from build123d import *

# Parameters (mm, degrees)
SKIZZE1_R                       = 32.5
SKIZZE1_R_2                     = 5
AUFSATZ_LINEAR_AUSTRAGEN1_DEPTH = 5
SCHNITT_LINEAR_AUSTRAGEN1_DEPTH = 6
KREISMUSTER1_COUNT              = 8


with BuildPart() as part:
    # Skizze1 → Aufsatz-Linear austragen1 (new body)
    with BuildSketch(Plane.XY):
        Circle(SKIZZE1_R)
        Circle(SKIZZE1_R_2, mode=Mode.SUBTRACT)
    extrude(amount=-AUFSATZ_LINEAR_AUSTRAGEN1_DEPTH)

    # Skizze2 → Schnitt-Linear austragen1 (cut, through all)
    with BuildSketch(Plane.XY):
        with BuildLine():
            Line((2.5, 27.386127875), (2.5, 9.682458366))
            ThreePointArc((2.5, 9.682458366), (3.826834324, 9.238795325), (5.078765016, 8.614298922))
            Line((5.078765016, 8.614298922), (17.597149778, 21.132683684))
            ThreePointArc((17.597149778, 21.132683684), (10.52379439, 25.406687144), (2.5, 27.386127875))
        make_face()
    schnitt_linear_austragen1 = extrude(amount=-SCHNITT_LINEAR_AUSTRAGEN1_DEPTH, mode=Mode.SUBTRACT)

    # Kreismuster1: Schnitt-Linear austragen1 ×8 about axis
    kreismuster1_axis = Axis((0, 0, 0), (0, 0, 1))
    for i in range(1, KREISMUSTER1_COUNT):
        add(schnitt_linear_austragen1.rotate(kreismuster1_axis, i * 360 / KREISMUSTER1_COUNT), mode=Mode.SUBTRACT)


solid = part.part
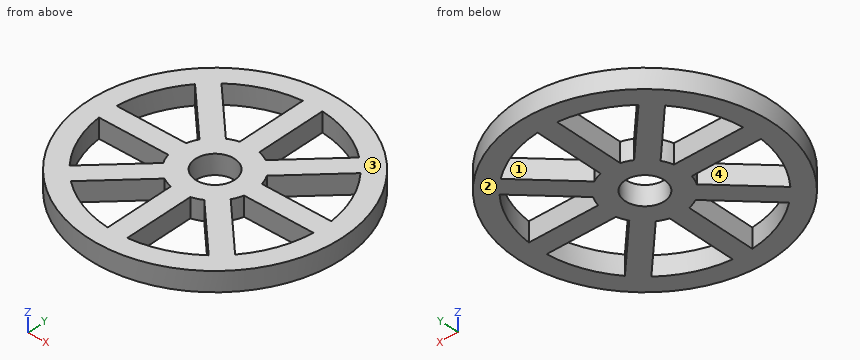
The listing builds one solid part. Answer for the finished solid, in the listing's coordinates (mm). Face numbers are marked on the shaded views. A direction names the side the tool comes from. Round coordinates to 2 decimals unless told otherwise and drop trailing zeros. Order: outer loops, then holes, each group sorted by start corner. A loop starts at its lowest first (then second) coordinate and runs counter-clockwise, first axis right, second up. Notation, with made-up numbers: (-35, 38.5) -> (-6, 38.5) arc R24 ccw to (-6, 64.5) -> close; hole circle Ø3 at (13, -8.5). An arc over 180 degrees is marked (long way). Write each question's results on one line, items separated by ' | '. Start each with the question number.
Q1. Find section D-D (x = 13.5). Determine the outline of the cut face in (y, z), then the cut area to 3 significant figures.
Q2. The mould has two halves that part along Y. Classify the marked faces 3 and 4: pulls with the +Y half, pulls with the -Y half, needs draft (parallel to the pull), parting line crosses it, or undercut.
Q3. Find section B-B (z = -3.9). Give the number of separate pieces and of enclosed holes in the cut face, then the cut area to 3 significant figures.
Q4. Straight lines are drawn through the part: probe 1 along Y at (x, z) = (22, -2.85); probe 2 along X at (y, z) = (-14, -0.65); probe 3 along Y at (x, z) = (0, -3.35). For each, find the intervals that lie inside material, in ascending order. Write a range as from..to.
Q5. Each of these flat-tipped pins is pushed along its axis until it touches: pin 1 (2.5 mm diameter, centred on y = -21, z = -1.5, fed in from +X); pin 2 (13 mm diameter, centred on x = 0, y = 0, fed in from +Z); pin 3 (1.5 mm diameter, centred on y = -6.5, z = -2.5, fed in from +X); pin 4 (1.5 mm diameter, centred on x = -17, z = -2, fed in from +Y). Where does it stop, or does it pass through?
Q6. Find section A-A (x = 0). Determine the outline of the cut face in (y, z).
Q7. Which of the six approach directions +Z, -Z, +X, -X, +Y, -Y give full straight-line access (tool end or side, diameter ignored) to the marked faces 1 and 2?
Worked answers:
1) outline: (-29.56, -5) -> (-23.96, -5) -> (-23.96, 0) -> (-29.56, 0) -> close; (-17.04, -5) -> (-9.96, -5) -> (-9.96, 0) -> (-17.04, 0) -> close; (-2.5, -5) -> (2.5, -5) -> (2.5, 0) -> (-2.5, 0) -> close; (9.96, -5) -> (17.04, -5) -> (17.04, 0) -> (9.96, 0) -> close; (23.96, -5) -> (29.56, -5) -> (29.56, 0) -> (23.96, 0) -> close | area: 152 mm2
2) face 3: needs draft | face 4: undercut
3) separate pieces: 1 | enclosed holes: 9 | area: 1,880 mm2
4) probe 1: y = -23.92..-16.5, -2.5..2.5, 16.5..23.92 | probe 2: x = -29.33..-23.67, -17.54..-10.46, -2.5..2.5, 10.46..17.54, 23.67..29.33 | probe 3: y = -32.5..-5, 5..32.5
5) pin 1: stops at x = 25.81 | pin 2: stops at z = 0 | pin 3: stops at x = 31.99 | pin 4: stops at y = 28.15
6) outline: (-32.5, -5) -> (-5, -5) -> (-5, 0) -> (-32.5, 0) -> close; (5, -5) -> (32.5, -5) -> (32.5, 0) -> (5, 0) -> close
7) face 1: +Z, -Z | face 2: -Z, +X, -X, +Y, -Y
